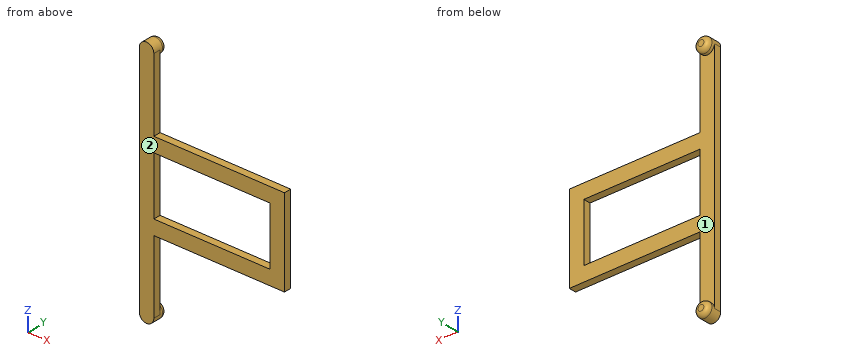
```python
from build123d import *

# Parameters (mm, degrees)
F0_DEPTH = 3.175
F1_R     = 3.175
F4_DEPTH = 6.35
F2_R     = 1.905


# Not quite as in the source:
# - a length typed as a fraction of an inch, garbled in the dataset ("3 / 203.2 mm" for 3/8 in), is restored


with BuildPart() as f0:
    # F3 (on Front) → F0 (new body)
    with BuildSketch(Plane.XZ):
        Polygon((6.35, 50.8), (0, 50.8), (0, 0), (0, -50.8), (6.35, -50.8), (6.35, -19.05), (63.5, -19.05), (63.5, 19.05), (6.35, 19.05), align=None)
        Polygon((6.35, -12.7), (6.35, 0), (6.35, 12.7), (57.15, 12.7), (57.15, -12.7), align=None, mode=Mode.SUBTRACT)
    extrude(amount=F0_DEPTH)

    # F1 (on face) → F4 (join)
    with BuildSketch(Plane.XZ.offset(3.175)):
        with Locations((3.175, -50.8)):
            Circle(F1_R)
        with Locations((3.175, 50.8)):
            Circle(F1_R)
    extrude(amount=-F4_DEPTH)

    # F2
    f2_edges = [f0.edges().sort_by_distance(p)[0] for p in [
        (0, 3.175, 50.8),
        (0, 3.175, -50.8),
    ]]
    fillet(f2_edges, radius=F2_R)


solid = f0.part
```
Source: CAD feature listing. Evaluate the final solid. Frame: model axes, mm. Face numbers are marked on the shaded views. Coordinates: 2 decimals unless noted, no trailing zeros. Loops run counter-clockwise (first coordinate to the right, second up) from the corner with the lowest first, then second, coordinate; pieces in that order, holes last. Notation, with made-up numbers: M 42,27 L 75,27 A27 cw 75,49 Z; hole C -32,74.25 d11. An arc over 180 degrees is marked long. Put each result on its own line as item: value. Start each with the question number.
1) Contact query for flat-ended pins moving along their axis: pin 1 Ø1 at (x, y) = (34, -1.5) entering from +Z; pin 2 Ø2.5 at (x, y) = (29.5, -1) entering from -Z; pin 3 Ø1 at (y, z) = (-1, -27.5) entering from +X; pin 4 Ø3.5 at (y, z) = (-2.5, -4.5) entering from -X. Output: stop coordinate, or through.
2) Cut plane A-A on x = 16. Return the cut outline in (y, z) (3 decimals).
3) Cut plane B-B on y = -1.75. Return the cut outline in (x, z) (3 decimals), then the cut area to 3 significant figures.
4) Ray query, L1, parallel to Z at x = 52.5, y = -3; L2, parallel to Z at x = 3, y = 0.5; L3, parallel to X at y = -2, z = 21. Return the intervals inside material, ascending. Write a range as from..to.
5) Pull-direction query (Z, two-part tool) for the marked faces 1 and 2; classes: pulls with the +Z half, pulls with the -Z half, needs draft (parallel to the pull), parting line crosses it, or undercut.
6) Cut plane C-C on z = 43. Return the cut outline in (x, y) (3 decimals), then the cut area to 3 significant figures.
The answers:
1. pin 1: stops at z = 19.05
1. pin 2: stops at z = -19.05
1. pin 3: stops at x = 6.35
1. pin 4: stops at x = 0
2. outline: M -3.175,-19.05 L 0,-19.05 L 0,-12.7 L -3.175,-12.7 Z; M -3.175,12.7 L 0,12.7 L 0,19.05 L -3.175,19.05 Z
3. outline: M 0,-50.8 A3.175 ccw 6.35,-50.8 L 6.35,-19.05 L 63.5,-19.05 L 63.5,19.05 L 6.35,19.05 L 6.35,50.8 A3.175 ccw 0,50.8 Z; hole M 6.35,-12.7 L 57.15,-12.7 L 57.15,12.7 L 6.35,12.7 Z
3. area: 1,560 mm²
4. L1: z = -19.05..-12.7, 12.7..19.05
4. L2: z = -53.97..-47.63, 47.63..53.97
4. L3: x = 0..6.35
5. face 1: undercut
5. face 2: needs draft
6. outline: M 0,-3.175 L 6.35,-3.175 L 6.35,0 L 0,0 Z
6. area: 20.2 mm²
